Part model, mm, in its own coordinate system. A direction names the side the tool comes from. Round coordinates to 2 decimals unless told otherwise and drop trailing zeros. Order: outer loops, then holes, each group sorted by start corner. A loop starts at its lowest first (then second) coordinate and runs counter-clockwise, first axis right, second up. Notation, with made-up numbers: (-22, 10.5) -> (5, 10.5) arc R16 ccw to (5, 20.5) -> close; hole circle Ø6 at (74, 88). An arc over 180 degrees is marked (long way). Return JSON: item names as keys, results as strings. Group by question number.
from build123d import *

# Parameters (mm, degrees)
EXTRUDE_1_DEPTH     = 210
SHELL_1_T           = 2
SKETCH_3_W          = 165
SKETCH_3_H          = 100
CUT_EXTRUDE_2_DEPTH = 2
EXTRUDE_2_DEPTH     = 6
CUT_EXTRUDE_3_DEPTH = 2
CUT_EXTRUDE_4_DEPTH = 2
CUT_EXTRUDE_5_DEPTH = 2
FILLET_1_R          = 1.5


with BuildPart() as part:
    # 草图2 → 凸台-拉伸1 (new body)
    with BuildSketch(Plane(origin=(0, 0, 0), x_dir=(0, 0, -1), z_dir=(1, 0, 0))):
        Polygon((0, 0), (0, 118.808397169), (109.625454917, 70), (109.625454917, 0), align=None)
    extrude(amount=EXTRUDE_1_DEPTH)

    # 抽壳1
    shell_1_openings = [part.faces().sort_by_distance(p)[0] for p in [
        (105, 0, -54.812727459),
    ]]
    offset(amount=SHELL_1_T, openings=shell_1_openings, kind=Kind.INTERSECTION)

    # 草图3 → 切除-拉伸2 (cut)
    with BuildSketch(Plane(origin=(0, 99.153366004, -44.14592279), x_dir=(1, 0, 0), z_dir=(0, 0.9135454576426035, -0.4067366430757946))):
        with Locations((105, 11.676271366)):
            Rectangle(SKETCH_3_W, SKETCH_3_H)
    extrude(amount=CUT_EXTRUDE_2_DEPTH, mode=Mode.SUBTRACT)

    # 草图5 → 凸台-拉伸2 (add)
    with BuildSketch(Plane(origin=(0, 99.153366004, -44.14592279), x_dir=(1, 0, 0), z_dir=(0, -0.9135454576426034, 0.4067366430757947))):
        Polygon((9.75, 43.073728634), (29.75, 43.073728634), (29.75, 41.073728634), (9.75, 41.073728634), (9.75, 21.073728634), (7.75, 21.073728634), (7.75, 43.073728634), align=None)
        Polygon((180.25, 43.073728634), (180.25, 41.073728634), (200.25, 41.073728634), (200.25, 21.073728634), (202.25, 21.073728634), (202.25, 43.073728634), (200.25, 43.073728634), align=None)
        Polygon((180.25, -66.426271366), (180.25, -64.426271366), (200.25, -64.426271366), (200.25, -44.426271366), (202.25, -44.426271366), (202.25, -66.426271366), (200.25, -66.426271366), align=None)
        Polygon((29.75, -66.426271366), (29.75, -64.426271366), (9.75, -64.426271366), (9.75, -44.426271366), (7.75, -44.426271366), (7.75, -66.426271366), (9.75, -66.426271366), align=None)
    extrude(amount=EXTRUDE_2_DEPTH)

    # 草图8 → 切除-拉伸3 (cut)
    with BuildSketch(Plane(origin=(0, 97.50898418, -43.413796832), x_dir=(-1, 0, 0), z_dir=(0, -0.9135454576426034, 0.4067366430757947))):
        Polygon((-19.75, -41.073728634), (-21.75, -43.073728634), (-19.75, -43.073728634), (-7.75, -31.073728634), (-7.75, -29.073728634), (-9.75, -31.073728634), align=None)
        Polygon((-19.75, 64.426271366), (-21.75, 66.426271366), (-19.75, 66.426271366), (-7.75, 54.426271366), (-7.75, 52.426271366), (-9.75, 54.426271366), align=None)
        Polygon((-190.25, -41.073728634), (-188.25, -43.073728634), (-190.25, -43.073728634), (-202.25, -31.073728634), (-202.25, -29.073728634), (-200.25, -31.073728634), align=None)
        Polygon((-200.25, 54.426271366), (-202.25, 52.426271366), (-202.25, 54.426271366), (-190.25, 66.426271366), (-188.25, 66.426271366), (-190.25, 64.426271366), align=None)
    extrude(amount=CUT_EXTRUDE_3_DEPTH, mode=Mode.SUBTRACT)

    # 草图10 → 切除-拉伸4 (cut)
    with BuildSketch(Plane.ZY.offset(2)):
        Polygon((-98.902140019, 61.638692052), (-9.521804093, 101.433381509), (-13.182433881, 109.655290628), (-102.562769807, 69.860601171), align=None)
    extrude(amount=-CUT_EXTRUDE_4_DEPTH, mode=Mode.SUBTRACT)

    # 草图11 → 切除-拉伸5 (cut)
    with BuildSketch(Plane(origin=(212, 0, 0), x_dir=(0, 0, -1), z_dir=(1, 0, 0))):
        Polygon((9.521804093, 101.433381509), (13.182433881, 109.655290628), (102.562769807, 69.860601171), (98.902140019, 61.638692052), align=None)
    extrude(amount=-CUT_EXTRUDE_5_DEPTH, mode=Mode.SUBTRACT)

    # 圆角1
    fillet_1_edges = [part.edges().sort_by_distance(p)[0] for p in [
        (212, 96.593471142, -54.812727459),
        (212, 60.944063548, 2),
        (-2, 60.944063548, 2),
        (-2, 96.593471142, -54.812727459),
        (-2, 35.649407593, -111.625454917),
        (105, 121.888127097, 2),
        (105, 71.298815186, -111.625454917),
        (212, 35.649407593, -111.625454917),
    ]]
    fillet(fillet_1_edges, radius=FILLET_1_R)


solid = part.part
(1) Mould opens along Z. For faces 1 (the cylindrical face through (-1.572, 96.255, -54.465)), 2 (the flat face through (190.11, 114.375, -5.962)), 3 (the flat face through (104, 59, 2)) say: pulls with the +Z half, pulls with the -Z half, needs draft (parallel to the pull), parting line crosses it, or undercut.
(2) Saw through at C-C, the plane x = 104.5. List the corners of the cut face in (y, z), and give its area (3 significant figures).
(3) Probe L1, parallel to X at y = 27, z = -29; L2, parallel to Z at x = 11.5, y = 15; L3, parallel to X at y = 110, z = -13.5. List the from-to ranges inside material, lowest first. Write a range as [from, to].
(4) Saw through at B-B, the plane y = 52.5. List the corners of the cut face in (x, z).
(5) Tool access for faces 4 (the flat face through (-1.014, 81.257, -54.838)), 5 (the flat face through (-1.014, 90.037, -57.247)), 6 (the flat face through (201.1, 69.5, -96)): list every direction of +Z, -Z, +X, -X, +Y, -Y with a clear straight run to the whole face (end or side of a thin tool).
(6) Saw through at A-A, the plane x = 183. List the corners of the cut face in (y, z).
(7) Saw through at D-D, the plane z = -72.5. State how many separate pieces and enclosed holes the cut face has, and give its area (3 significant figures).
(8) Pin check, flat tips, straight feed: P1, Ø15, axis at y = 108, z = -14, coming from the +X side; P2, Ø5, axis at x = 188.5, z = -43.5, coming from the +Y side; P3, Ø8, axis at y = 98.5, z = -27.5, coming from the +X side. Stop position of each tip, or through.
Results are:
{
 "1": {"face 1": "pulls with the -Z half", "face 2": "undercut", "face 3": "pulls with the +Z half"},
 "2": {"outline": "(0, -111.63) -> (70.32, -111.63) arc R1.5 ccw to (71.7, -110.74) -> (75.89, -101.3) -> (74.07, -100.49) -> (70, -109.63) -> (0, -109.63) -> close; (0, 0) -> (118.81, 0) -> (114.74, -9.14) -> (116.57, -9.95) -> (120.95, -0.11) arc R1.5 ccw to (119.58, 2) -> (0, 2) -> close", "area": "425 mm^2"},
 "3": {"L1": "x = [-2, 0], [210, 212]", "L2": "z = [-111.63, -109.63], [0, 2]", "L3": "x = [-2, 0], [7.75, 9.08], [200.92, 202.25], [210, 212]"},
 "4": {"outline": "(-2, -110.13) arc R1.5 ccw to (-0.5, -111.63) -> (210.5, -111.63) arc R1.5 ccw to (212, -110.13) -> (212, 0.5) arc R1.5 ccw to (210.5, 2) -> (-0.5, 2) arc R1.5 ccw to (-2, 0.5) -> close; hole (0, -109.63) -> (210, -109.63) -> (210, 0) -> (0, 0) -> close"},
 "5": {"face 4": "+X, -X", "face 5": "-X", "face 6": "-Y"},
 "6": {"outline": "(0, -111.63) -> (70.32, -111.63) arc R1.5 ccw to (71.7, -110.74) -> (75.89, -101.3) -> (74.07, -100.49) -> (72.95, -103) -> (67.47, -100.56) -> (66.65, -102.39) -> (72.14, -104.83) -> (70, -109.63) -> (0, -109.63) -> close; (0, 0) -> (118.81, 0) -> (116.67, -4.8) -> (111.19, -2.36) -> (110.38, -4.18) -> (115.86, -6.62) -> (114.74, -9.14) -> (116.57, -9.95) -> (120.95, -0.11) arc R1.5 ccw to (119.58, 2) -> (0, 2) -> close"},
 "7": {"separate pieces": "4", "enclosed holes": "0", "area": "413 mm^2"},
 "8": {"P1": "stops at x = 212", "P2": "stops at y = 102.74", "P3": "passes through"}
}
